```python
from build123d import *

# Parameters (mm, degrees)
SKETCH1_R           = 2.286
BOSS_EXTRUDE1_DEPTH = 1.5875
FILLET1_R           = 4.7625


with BuildPart() as part:
    # Sketch1 → Boss-Extrude1 (new body)
    with BuildSketch(Plane.XY):
        Polygon((-17.4625, 0), (17.4625, 0), (17.4625, 9.525), (0, 49.2125), (-17.4625, 9.525), align=None)
        with Locations((-12.7, 4.7625)):
            Circle(SKETCH1_R, mode=Mode.SUBTRACT)
        with Locations((12.7, 4.7625)):
            Circle(SKETCH1_R, mode=Mode.SUBTRACT)
    extrude(amount=BOSS_EXTRUDE1_DEPTH)

    # Fillet1
    fillet1_edges = [part.edges().sort_by_distance(p)[0] for p in [
        (17.4625, 0, 0.79375),
        (-17.4625, 0, 0.79375),
        (-17.4625, 9.525, 0.79375),
        (0, 49.2125, 0.79375),
        (17.4625, 9.525, 0.79375),
    ]]
    fillet(fillet1_edges, radius=FILLET1_R)


solid = part.part
```
The model under review builds one solid part; all positions refer to its coordinate system, in mm. Give positions to 0.01 mm unless a question says otherwise; leave off trailing zeros. Write each loop counter-clockwise with the first axis right and the second up, starting at its lowest first coordinate (ties: lowest second). Pieces come first, ordered by that corner, then holes. Notation, with made-up numbers: (86.5, -22.5) - (105.5, -22.5) arc R38 cw to (105.5, 15.5) - close; hole circle Ø3 at (52, 13.25). An arc over 180 degrees is marked (long way). Answer in a Markdown table with one row per item. Add a question column.
1. Insertion check: P1, Ø2.5, axis at x = 12.7, y = 4.76, coming from the +Z side; P2, Ø1, axis at x = 8, y = 22, coming from the -Z side. Each pin has a flat end and moves straight along its axis. Give the tip position at first contact, or say it passes through.
2. Wall thickness on line 1 along Y through (x, z) = (-12.7, 0.7); line 2 along X through (y, z) = (21, 0.6); line 3 along X through (y, z) = (26.5, 0.55): over which ranges is each line inside the solid? List them lowest first. Write a range as [from, to].
3. We need section D-D on y = 29.5. Write out the cut boundary in (x, z).
4. We need section C-C on x = -5.5. Write out the cut boundary in (y, z).
5. We need section B-B on x = -11. Write out the cut boundary in (y, z), then the cut area to 3 significant figures.
6. Draft analysis for pull direction X (two halves, no side actions). For faces 1 (the cylindrical face through (13.75, 2.73, 0.78)), 2 (the flat face through (0, 0, 1)), 3 (the flat face through (10.8, 24.67, 0.78)), state which applies: +X half, -X half, draft (parallel to the pull), parting line (faces both ways), or undercut.
7. We need section A-A on z = 1. Write out the cut boundary in (x, y) (1 decimal), then the cut area to 3 significant figures.
Ans:
| question | item | result |
|---|---|---|
| 1 | P1 | passes through |
| 1 | P2 | stops at z = 0 |
| 2 | line 1 | y = [0, 2.48], [7.05, 20.35] |
| 2 | line 2 | x = [-12.41, 12.41] |
| 2 | line 3 | x = [-9.99, 9.99] |
| 3 | outline | (-8.67, 0) - (8.67, 0) - (8.67, 1.59) - (-8.67, 1.59) - close |
| 4 | outline | (0, 0) - (36.71, 0) - (36.71, 1.59) - (0, 1.59) - close |
| 5 | outline | (0, 0) - (3.23, 0) - (3.23, 1.59) - (0, 1.59) - close; (6.29, 0) - (24.21, 0) - (24.21, 1.59) - (6.29, 1.59) - close |
| 5 | area | 33.6 mm^2 |
| 6 | face 1 | undercut |
| 6 | face 2 | draft |
| 6 | face 3 | +X half |
| 7 | outline | (-17.5, 4.8) arc R4.8 ccw to (-12.7, 0) - (12.7, 0) arc R4.8 ccw to (17.5, 4.8) - (17.5, 8.5) arc R4.8 ccw to (17.1, 10.4) - (4.4, 39.3) arc R4.8 ccw to (-4.4, 39.3) - (-17.1, 10.4) arc R4.8 ccw to (-17.5, 8.5) - close; hole circle Ø4.6 at (-12.7, 4.8); hole circle Ø4.6 at (12.7, 4.8) |
| 7 | area | 958 mm^2 |
